```python
from build123d import *

# Parameters (mm, degrees)
SKETCH1_W                    = 1343.025
SKETCH1_H                    = 527.05
BOSS_EXTRUDE1_DEPTH          = 17.78
FILLET1_R                    = 6.35
SKETCH5_W                    = 152.4
SKETCH5_H                    = 400.05
CUT_EXTRUDE1_DEPTH           = 18.78
F_1_8_0_125_DIAMETER_HOLE2_D = 3.175
CUT_EXTRUDE2_DEPTH           = 18.78
FILLET2_R                    = 6.35


with BuildPart() as part:
    # Sketch1 → Boss-Extrude1 (new body)
    with BuildSketch(Plane(origin=(0, 0, 0), x_dir=(1, 0, 0), z_dir=(0, 1, 0))):
        Rectangle(SKETCH1_W, SKETCH1_H)
    extrude(amount=BOSS_EXTRUDE1_DEPTH)

    # Fillet1
    fillet1_edges = [part.edges().sort_by_distance(p)[0] for p in [
        (671.5125, 8.89, 263.525),
        (-671.5125, 8.89, 263.525),
        (-671.5125, 8.89, -263.525),
        (671.5125, 8.89, -263.525),
    ]]
    fillet(fillet1_edges, radius=FILLET1_R)

    # Sketch5 → Cut-Extrude1 (cut, through all)
    with BuildSketch(Plane(origin=(0, 17.78, 0), x_dir=(1, 0, 0), z_dir=(0, 1, 0))):
        Polygon((-406.4, 200.025), (406.4, 200.025), (0, 38.1), align=None)
        Polygon((0, -38.1), (-406.4, -200.025), (406.4, -200.025), align=None)
        Polygon((406.4, 146.74453125), (406.4, -146.74453125), (38.1, 0), align=None)
        Polygon((-406.4, 146.74453125), (-38.1, 0), (-406.4, -146.74453125), align=None)
        with Locations((550.8625, 0)):
            Rectangle(SKETCH5_W, SKETCH5_H)
        with Locations((-550.8625, 0)):
            Rectangle(SKETCH5_W, SKETCH5_H)
    extrude(amount=-CUT_EXTRUDE1_DEPTH, mode=Mode.SUBTRACT)

    # 1/8 (0.125) Diameter Hole2 (through all)
    with Locations(Plane(origin=(0, 17.78, 0), x_dir=(1, 0, 0), z_dir=(0, 1, 0))):
        with Locations((0, 0), (-439.865615282, -175.258956089), (439.865615282, 175.258956089), (439.865615282, -175.258956089), (-439.865615282, 175.258956089)):
            Hole(F_1_8_0_125_DIAMETER_HOLE2_D / 2)

    # Sketch8 → Cut-Extrude2 (cut, through all)
    with BuildSketch(Plane(origin=(0, 17.78, 0), x_dir=(1, 0, 0), z_dir=(0, 1, 0))):
        with BuildLine():
            Line((-82.55, -263.525), (-82.55, -234.95))
            ThreePointArc((-82.55, -234.95), (-80.690128061, -230.459871939), (-76.2, -228.6))
            Line((-76.2, -228.6), (76.2, -228.6))
            ThreePointArc((76.2, -228.6), (80.690128061, -230.459871939), (82.55, -234.95))
            Line((82.55, -234.95), (82.55, -263.525))
            Line((82.55, -263.525), (-82.55, -263.525))
        make_face()
    extrude(amount=-CUT_EXTRUDE2_DEPTH, mode=Mode.SUBTRACT)

    # Fillet2
    fillet2_edges = [part.edges().sort_by_distance(p)[0] for p in [
        (82.55, 8.89, 263.525),
        (-82.55, 8.89, 263.525),
        (406.4, 8.89, -200.025),
        (0, 8.89, -38.1),
        (-406.4, 8.89, -200.025),
        (-474.6625, 8.89, -200.025),
        (-474.6625, 8.89, 200.025),
        (-627.0625, 8.89, 200.025),
        (-627.0625, 8.89, -200.025),
        (-406.4, 8.89, 146.74453125),
        (-406.4, 8.89, -146.74453125),
        (-38.1, 8.89, 0),
        (627.0625, 8.89, -200.025),
        (627.0625, 8.89, 200.025),
        (474.6625, 8.89, 200.025),
        (474.6625, 8.89, -200.025),
        (0, 8.89, 38.1),
        (406.4, 8.89, 200.025),
        (-406.4, 8.89, 200.025),
        (38.1, 8.89, 0),
        (406.4, 8.89, -146.74453125),
        (406.4, 8.89, 146.74453125),
    ]]
    fillet(fillet2_edges, radius=FILLET2_R)


solid = part.part
```
Work out the finished part from the listing and answer in its coordinate system (mm). A direction names the side the tool comes from. Coordinates: 2 decimals unless noted, no trailing zeros. Order: outer loops, then holes, each group sorted by start corner. A loop starts at its lowest first (then second) coordinate and runs counter-clockwise, first axis right, second up. Notation, with made-up numbers: (-8.5, 6) - (11.5, 6) arc R26 cw to (11.5, 26) - close; hole circle Ø4 at (88, 84). An arc over 180 degrees is marked (long way). Answer as a JSON object with one key per item and string values.
1. Find section A-A on x = -575. Determine the outline of the cut face in (y, z) (3 decimals).
Output values:
{"outline": "(0, -263.525) - (17.78, -263.525) - (17.78, -200.025) - (0, -200.025) - close; (0, 200.025) - (17.78, 200.025) - (17.78, 263.525) - (0, 263.525) - close"}
2. Find section C-C on z = 72. Determine the outline of the cut face in (x, y).
Output values:
{"outline": "(-671.51, 0) - (-627.06, 0) - (-627.06, 17.78) - (-671.51, 17.78) - close; (-474.66, 0) - (-406.4, 0) - (-406.4, 17.78) - (-474.66, 17.78) - close; (-218.81, 0) - (-85.08, 0) - (-85.08, 17.78) - (-218.81, 17.78) - close; (85.08, 0) - (218.81, 0) - (218.81, 17.78) - (85.08, 17.78) - close; (406.4, 0) - (474.66, 0) - (474.66, 17.78) - (406.4, 17.78) - close; (627.06, 0) - (671.51, 0) - (671.51, 17.78) - (627.06, 17.78) - close"}
3. A tool of negligible diameter and unlimited length cuts with its end or side. For faces 1 (the face through (-9, 17.78, -4)), 2 (the face through (-186.391, 9.014, -112.365)), from which of +Z, -Z, +X, -X, +Y, -Y can it reach the whole face along a straight path? Write none if from no direction.
Output values:
{"face 1": "+Z, -Z, +X, -X, +Y", "face 2": "+Y, -Y"}
4. The mould has two halves that part along X. Classify faces 3 (the face through (191.62, 9.01, -114.45)), 4 (the face through (-186.391, 9.014, 112.365)), 5 (the face through (-9, 0, -4)): +X half, -X half, draft (parallel to the pull), parting line (faces both ways), or undercut.
Output values:
{"face 3": "undercut", "face 4": "undercut", "face 5": "draft"}
5. Consider line 1 (Z direction, x = 50.5, y = 9.25) (3 decimals); line 2 (Z direction, x = 397, y = 10) (3 decimals); line 3 (Z direction, x = 17, y = 11) (3 decimals). Determine where each line is inside the solid, lowest interval first.
Output values:
{"line 1": "z = -263.525 to -200.025, -58.221 to -4.208, 4.208 to 58.221, 200.025 to 228.6", "line 2": "z = -263.525 to -142.999, 142.999 to 263.525", "line 3": "z = -263.525 to -200.025, -44.873 to 44.873, 200.025 to 228.6"}
6. Find section D-D on y = 3. Count the separate pieces of the cut face and the enclosed holes in it, plus the area to 3 significant figures.
Output values:
{"separate pieces": "1", "enclosed holes": "11", "area": "341,000 mm²"}
7. This flat-tipped pin is pushed along its axis until it touches: P1, Ø1, axis at x = 57, y = 15.5, coming from the +Z side. Where does it stop, or does it pass through?
Output values:
{"P1": "stops at z = 228.6"}
8. Find section B-B on x = 296.5. Determine the outline of the cut face in (y, z) (3 decimals).
Output values:
{"outline": "(0, -263.525) - (17.78, -263.525) - (17.78, -200.025) - (0, -200.025) - close; (0, -156.237) - (17.78, -156.237) - (17.78, -102.956) - (0, -102.956) - close; (0, 102.956) - (17.78, 102.956) - (17.78, 156.237) - (0, 156.237) - close; (0, 200.025) - (17.78, 200.025) - (17.78, 263.525) - (0, 263.525) - close"}
